Autodesk Inventor part; units mm, degrees
ref_plane "YZ Plane" through (0, 0, 0) normal (1, 0, 0) x (0, 1, 0)
ref_plane "XZ Plane" through (0, 0, 0) normal (0, 1, 0) x (-1, 0, 0)
ref_plane "XY Plane" through (0, 0, 0) normal (0, 0, 1) x (1, 0, 0)
sketch "Sketch1" plane through (0, 0, 0) normal (0, 1, 0) x (-1, 0, 0)
  line L0 (10.35, 0) -> (-10.35, 0)
  line L1 (-10.35, 0) -> (-10.35, 41.3)
  line L2 (-10.35, 41.3) -> (10.35, 41.3)
  line L3 (10.35, 41.3) -> (10.35, 0)
  point P0 (0, 0)
  point P1 (0, 0)
  dimension "d0" = 41.3
  dimension "d1" = 20.7
extrude "Extrusion1" add sketch "Sketch1" against normal blind 40.2
ref_plane "Work Plane2" through (0, -8.6, 0) normal (0, -1, 0) x (1, 0, 0)
ref_plane "Work Plane1" through (0, 5.9, 0) normal (0, -1, 0) x (1, 0, 0)
sketch "Sketch2" plane through (0, -8.6, 0) normal (0, -1, 0) x (1, 0, 0)
  line L0 (-10.35, 0) -> (10.35, 0)
  line L1 (-10.35, 41.3) -> (-10.35, 0) construction
  line L2 (-10.35, 0) -> (-10.35, -7.3)
  line L3 (-10.35, -7.3) -> (-6.25, -7.3)
  arc A0 (-6.25, -7.3) -> (-6.0496, -6.4902) centre (-6.25, -6.8703) ccw
  arc A1 (-3.9504, -6.4902) -> (-6.0496, -6.4902) centre (-5, -4.5) ccw
  arc A2 (-3.9504, -6.4902) -> (-3.75, -7.3) centre (-3.75, -6.8703) ccw
  line L4 (-3.75, -7.3) -> (0, -7.3)
  line L5 (0, -7.3) -> (0, 0) construction
  line L6 (10.35, 0) -> (10.35, -7.3)
  line L7 (10.35, -7.3) -> (6.25, -7.3)
  arc A3 (6.0496, -6.4902) -> (6.25, -7.3) centre (6.25, -6.8703) ccw
  arc A4 (6.0496, -6.4902) -> (3.9504, -6.4902) centre (5, -4.5) ccw
  arc A5 (3.75, -7.3) -> (3.9504, -6.4902) centre (3.75, -6.8703) ccw
  line L8 (3.75, -7.3) -> (0, -7.3)
  line L9 (-10.35, 20.65) -> (10.35, 20.65) construction
  line L10 (10.35, 0) -> (10.35, 41.3) construction
  line L11 (-10.35, 41.3) -> (10.35, 41.3)
  line L12 (-10.35, 41.3) -> (-10.35, 48.6)
  line L13 (-10.35, 48.6) -> (-6.25, 48.6)
  arc A6 (-6.0496, 47.7902) -> (-6.25, 48.6) centre (-6.25, 48.1703) ccw
  arc A7 (-6.0496, 47.7902) -> (-3.9504, 47.7902) centre (-5, 45.8) ccw
  arc A8 (-3.75, 48.6) -> (-3.9504, 47.7902) centre (-3.75, 48.1703) ccw
  line L14 (-3.75, 48.6) -> (0, 48.6)
  line L15 (0, 48.6) -> (0, 41.3) construction
  line L16 (10.35, 48.6) -> (6.25, 48.6)
  arc A9 (6.25, 48.6) -> (6.0496, 47.7902) centre (6.25, 48.1703) ccw
  arc A10 (3.9504, 47.7902) -> (6.0496, 47.7902) centre (5, 45.8) ccw
  arc A11 (3.9504, 47.7902) -> (3.75, 48.6) centre (3.75, 48.1703) ccw
  line L17 (3.75, 48.6) -> (0, 48.6)
  line L18 (10.35, 41.3) -> (10.35, 48.6)
  dimension "d7" = 4.5
  dimension "d8" = 10
  dimension "d9" = 55.9
  dimension "d10" = 50.3
  dimension "d11" = 2.5
extrude "Extrusion2" add sketch "Sketch2" along normal blind 2
sketch "Sketch3" plane through (0, 5.9, 0) normal (0, -1, 0) x (1, 0, 0)
  circle A0 centre (0, 10.7) radius 2.5
  arc A1 (-3.9504, -6.4902) -> (-6.0496, -6.4902) centre (-5, -4.5) ccw construction
  point P0 (0, 0)
  dimension "d17" = 5
  dimension "d18" = 15.2
extrude "Extrusion3" add sketch "Sketch3" along normal up to next
properties part number "SM-S4303R"
Input: part model. Units: mm. Frame: model coordinates. A direction names the side the tool comes from. Coordinates: 2 decimals unless noted, no trailing zeros. Write each loop counter-clockwise with the first axis right and the second up, starting at its lowest first coordinate (ties: lowest second). Pieces come first, ordered by that corner, then holes.
1) Section C-C on z = 10.7. Output: boundary loops of the cut face in (x, y).
2) Mould query, pull axis X, two halves, no side actions, for faces 1 (the flat face through (0, 0, 21)), 2 (the cylindrical face through (-0.33, 2.99, 8.22)), 3 (the cylindrical face through (4.92, -9.59, -2.25)). Classes: pulls with the +X half, pulls with the -X half, needs draft (parallel to the pull), parting line crosses it, or undercut.
3) Pin query (flat end, axial travel): pin 1 Ø4.5 at (x, y) = (-3.5, -2.5) entering from -Z; pin 2 Ø8 at (x, z) = (0, 45.5) entering from +Y; pin 3 Ø2 at (x, z) = (1.5, 46) entering from -Y; pin 4 Ø3.5 at (x, z) = (-5, -4.5) entering from -Y (1 decimal). Return the tip coordinate at first contact, or that it passes through.
4) Set-up query: faces 4 (the flat face through (0, -25, 0)), 5 (the flat face through (0, -4, 0)), 6 (the flat face through (0, -8.6, 45)), 7 (the flat face through (0, -10.6, 45)). Return all of +Z, -Z, +X, -X, +Y, -Y with unobstructed straight access to the full face (end or side cutting, diameter ignored); none if empty.
5) Section A-A on z = 45.8. Output: boundary loops of the cut face in (x, y).
6) Section D-D on y = -15. Output: boundary loops of the cut face in (x, z).
7) Section B-B on x = -5. Output: boundary loops of the cut face in (y, z).
8) Material intervals for line 1 along X through (y, z) = (-9.7, 45.8); line 2 along Y through (x, z) = (3.5, 34); line 3 along Z through (x, y) = (-7.25, -12.5), sorted ascending.
Check result:
1. outline: (-10.35, -40.2) - (10.35, -40.2) - (10.35, 0) - (2.5, 0) - (2.5, 5.9) - (-2.5, 5.9) - (-2.5, 0) - (-10.35, 0) - close
2. face 1: needs draft
2. face 2: parting line crosses it
2. face 3: undercut
3. pin 1: stops at z = 0
3. pin 2: stops at y = -8.6
3. pin 3: stops at y = -10.6
3. pin 4: passes through
4. face 4: -Z, +X, -X, -Y
4. face 5: -Z, +X, -X, +Y
4. face 6: +Z, +X, -X, +Y
4. face 7: +Z, +X, -X, -Y
5. outline: (-10.35, -10.6) - (-7.25, -10.6) - (-7.25, -8.6) - (-10.35, -8.6) - close; (-2.75, -10.6) - (2.75, -10.6) - (2.75, -8.6) - (-2.75, -8.6) - close; (7.25, -10.6) - (10.35, -10.6) - (10.35, -8.6) - (7.25, -8.6) - close
6. outline: (-10.35, 0) - (10.35, 0) - (10.35, 41.3) - (-10.35, 41.3) - close
7. outline: (-40.2, 0) - (-10.6, 0) - (-10.6, -2.25) - (-8.6, -2.25) - (-8.6, 0) - (0, 0) - (0, 41.3) - (-8.6, 41.3) - (-8.6, 43.55) - (-10.6, 43.55) - (-10.6, 41.3) - (-40.2, 41.3) - close
8. line 1: x = -10.35 to -7.25, -2.75 to 2.75, 7.25 to 10.35
8. line 2: y = -40.2 to 0
8. line 3: z = 0 to 41.3
